Geometry check sheet. Reference: the model listing, model coordinates, mm. Face numbers are marked on the shaded views. A direction names the side the tool comes from. Round coordinates to 2 decimals unless told otherwise and drop trailing zeros. Loops run counter-clockwise (first coordinate to the right, second up) from the corner with the lowest first, then second, coordinate; pieces in that order, holes last.
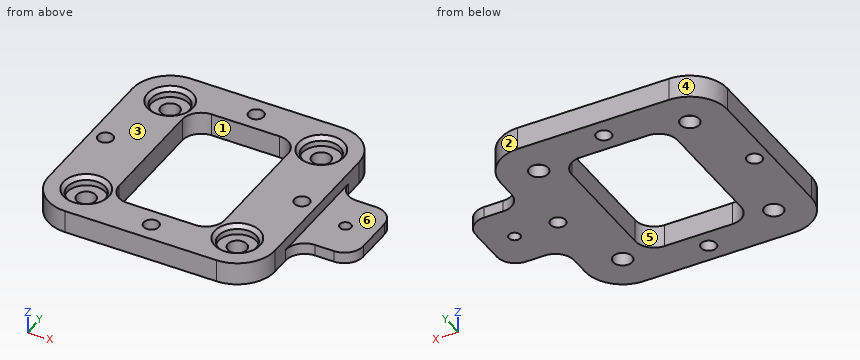
```python
from build123d import *

# Parameters (mm, degrees)
F0_R     = 5
F0_R_2   = 2
F0_W     = 28
F0_H     = 40.175457
F1_DEPTH = 6
F0_R_3   = 2.5
F2_DEPTH = 3.5
F0_W_2   = 15
F0_H_2   = 20
F0_R_4   = 1.5
F3_DEPTH = 3
F4_R     = 10
F5_R     = 5
F6_SIZE  = 1


with BuildPart() as f1:
    # F0 (on Top) → F1 (new body)
    with BuildSketch(Plane.XY):
        Polygon((-28.548011, 39.848171), (-88.548011, 39.848171), (-88.548011, -20.151829), (-28.548011, -20.151829), (-28.548011, -0.151829), (-28.548011, 19.848171), align=None)
        with Locations((-78.548011, -10.151829)):
            Circle(F0_R, mode=Mode.SUBTRACT)
        with Locations((-58.548011, -15.151829)):
            Circle(F0_R_2, mode=Mode.SUBTRACT)
        with Locations((-84.548011, 9.848171)):
            Circle(F0_R_2, mode=Mode.SUBTRACT)
        with Locations((-58.548011, 9.760442)):
            Rectangle(F0_W, F0_H, mode=Mode.SUBTRACT)
        with Locations((-38.548011, -10.151829)):
            Circle(F0_R, mode=Mode.SUBTRACT)
        with Locations((-78.548011, 29.848171)):
            Circle(F0_R, mode=Mode.SUBTRACT)
        with Locations((-58.548011, 34.848171)):
            Circle(F0_R_2, mode=Mode.SUBTRACT)
        with Locations((-32.548011, 9.848171)):
            Circle(F0_R_2, mode=Mode.SUBTRACT)
        with Locations((-38.548011, 29.848171)):
            Circle(F0_R, mode=Mode.SUBTRACT)
    extrude(amount=F1_DEPTH)

    # F0 (on Top) → F2 (join)
    with BuildSketch(Plane.XY):
        with Locations((-78.548011, 29.848171)):
            Circle(F0_R)
        with Locations((-78.548011, 29.848171)):
            Circle(F0_R_3, mode=Mode.SUBTRACT)
        with Locations((-78.548011, -10.151829)):
            Circle(F0_R)
        with Locations((-78.548011, -10.151829)):
            Circle(F0_R_3, mode=Mode.SUBTRACT)
        with Locations((-38.548011, 29.848171)):
            Circle(F0_R)
        with Locations((-38.548011, 29.848171)):
            Circle(F0_R_3, mode=Mode.SUBTRACT)
        with Locations((-38.548011, -10.151829)):
            Circle(F0_R)
        with Locations((-38.548011, -10.151829)):
            Circle(F0_R_3, mode=Mode.SUBTRACT)
    extrude(amount=F2_DEPTH)

    # F0 (on Top) → F3 (join)
    with BuildSketch(Plane.XY):
        with Locations((-21.048011, 9.848171)):
            Rectangle(F0_W_2, F0_H_2)
        with Locations((-21.048011, 9.848171)):
            Circle(F0_R_4, mode=Mode.SUBTRACT)
    extrude(amount=F3_DEPTH)

    # F4
    f4_edges = [f1.edges().sort_by_distance(p)[0] for p in [
        (-88.548011, 39.848171, 3),
        (-88.548011, -20.151829, 3),
        (-28.548011, -20.151829, 3),
        (-28.548011, 39.848171, 3),
    ]]
    fillet(f4_edges, radius=F4_R)

    # F5
    f5_edges = [f1.edges().sort_by_distance(p)[0] for p in [
        (-44.548011, 29.848171, 3),
        (-72.548011, 29.848171, 3),
        (-72.548011, -10.327286, 3),
        (-44.548011, -10.327286, 3),
        (-28.548011, -0.151829, 1.5),
        (-28.548011, 19.848171, 1.5),
        (-13.548011, -0.151829, 1.5),
        (-13.548011, 19.848171, 1.5),
    ]]
    fillet(f5_edges, radius=F5_R)

    # F6
    f6_edges = [f1.edges().sort_by_distance(p)[0] for p in [
        (-83.548011, 29.848171, 6),
        (-83.548011, -10.151829, 6),
        (-43.548011, 29.848171, 6),
        (-43.548011, -10.151829, 6),
    ]]
    chamfer(f6_edges, length=F6_SIZE)


solid = f1.part
```
1) Gauge pin test, flat ends, axial feed: pin 1 (7.5 mm diameter, centred on x = -18, y = 11, fed in from +Z); pin 2 (1.5 mm diameter, centred on x = -21, z = 1.5, fed in from -Y); pin 3 (1.5 mm diameter, centred on x = -21, z = 1, fed in from +Y); pin 4 (13 mm diameter, centred on x = -38.55, y = -10.15, fed in from -Z). Record the tip position at first contact, or that the pin passes through.
Report:
pin 1: stops at z = 3
pin 2: stops at y = -0.15
pin 3: stops at y = 19.85
pin 4: stops at z = 0
2) Sectioned sample at C-C, the plane z = 1.5. State how many separate pieces and enclosed holes the cut face has, then the cut area to 3 significant figures.
Report:
separate pieces: 1
enclosed holes: 10
area: 2,570 mm2
3) Sectioned sample at A-A, the plane y = 7. Record the cut outline in (x, z).
Report:
outline: (-88.55, 0) - (-72.55, 0) - (-72.55, 6) - (-88.55, 6) - close; (-44.55, 0) - (-13.55, 0) - (-13.55, 3) - (-28.55, 3) - (-28.55, 6) - (-44.55, 6) - close
4) Sectioned sample at D-D, the plane x = -71. Record the cut outline in (y, z), then the cut area to 3 significant figures.
Report:
outline: (-20.15, 0) - (-8.94, 0) - (-8.94, 6) - (-20.15, 6) - close; (28.47, 0) - (39.85, 0) - (39.85, 6) - (28.47, 6) - close
area: 136 mm2
5) Mould release check, pull along X, two halves, no side actions. Record for the marked faces 1, 2 and 3: +X half, -X half, draft (parallel to the pull), parting line (faces both ways), or undercut.
Report:
face 1: undercut
face 2: +X half
face 3: draft
6) Scan lines: line 1 along Y through (x, z) = (-78.5, 4.75); line 2 along X through (y, z) = (12, 2.3); line 3 along Y through (x, z) = (-55.5, 0.3). Record each from-to range of solid material in increasing order.
Report:
line 1: y = -20.15 to -15.15, -5.15 to 24.85, 34.85 to 39.85
line 2: x = -88.55 to -72.55, -44.55 to -13.55
line 3: y = -20.15 to -10.33, 29.85 to 39.85
7) Sectioned sample at B-B, the plane x = -52.5. Record the cut outline in (y, z).
Report:
outline: (-20.15, 0) - (-10.33, 0) - (-10.33, 6) - (-20.15, 6) - close; (29.85, 0) - (39.85, 0) - (39.85, 6) - (29.85, 6) - close
8) Access from +Z, -Z, +X, -X, +Y, -Y to the whole of each face (thin tool, end or side, straight path). Record for the marked faces 4, 5 and 6.
Report:
face 4: +Z, -Z, -X, +Y
face 5: +Z, -Z
face 6: +Z, +X, +Y, -Y
